Check sheet for the modelled part. Datum: model origin and axes. Units: mm. A direction names the side the tool comes from. Give positions to 0.01 mm unless a question says otherwise; leave off trailing zeros. Order: outer loops, then holes, each group sorted by start corner. A loop starts at its lowest first (then second) coordinate and runs counter-clockwise, first axis right, second up.
from build123d import *

# Parameters (mm, degrees)
SKETCH1_R           = 2
BOSS_EXTRUDE1_DEPTH = 10
CHAMFER2_SIZE       = 10
BOSS_EXTRUDE2_DEPTH = 10
BOSS_EXTRUDE3_DEPTH = 10
SKETCH6_W           = 239.348674296
SKETCH6_H           = 140
BOSS_EXTRUDE4_DEPTH = 10
CUT_EXTRUDE1_DEPTH  = 10
CUT_EXTRUDE2_DEPTH  = 10
CUT_EXTRUDE3_DEPTH  = 10
BOSS_EXTRUDE5_DEPTH = 40
SKETCH13_R          = 10
CUT_EXTRUDE4_DEPTH  = 15
BOSS_EXTRUDE6_DEPTH = 40
SKETCH15_R          = 10
CUT_EXTRUDE5_DEPTH  = 15
BOSS_EXTRUDE7_DEPTH = 40
SKETCH17_R          = 10
CUT_EXTRUDE6_DEPTH  = 15


with BuildPart() as part:
    # Sketch1 → Boss-Extrude1 (new body)
    with BuildSketch(Plane(origin=(0, 0, 0), x_dir=(1, 0, 0), z_dir=(0, 1, 0))):
        Polygon((0, 181.282032303), (-136.994845224, -56), (136.994845224, -56), align=None)
        with Locations(Location((-38.248711306, 59.033320997, 0), (0, 0, 270))):
            Circle(SKETCH1_R, mode=Mode.SUBTRACT)
        with Locations(Location((-50.748711306, 37.382685902, 0), (0, 0, 270))):
            Circle(SKETCH1_R, mode=Mode.SUBTRACT)
        with Locations(Location((37.748711306, 59.899346401, 0), (0, 0, 270))):
            Circle(SKETCH1_R, mode=Mode.SUBTRACT)
        with Locations(Location((50.248711306, 38.248711306, 0), (0, 0, 270))):
            Circle(SKETCH1_R, mode=Mode.SUBTRACT)
        with Locations(Location((-12, -28, 0), (0, 0, 270))):
            Circle(SKETCH1_R, mode=Mode.SUBTRACT)
        with Locations(Location((13, -28, 0), (0, 0, 270))):
            Circle(SKETCH1_R, mode=Mode.SUBTRACT)
    extrude(amount=BOSS_EXTRUDE1_DEPTH)

    # Chamfer2
    chamfer2_edges = [part.edges().sort_by_distance(p)[0] for p in [
        (68.497422612, 0, -62.641016151),
        (-68.497422612, 0, -62.641016151),
        (0, 0, 56),
    ]]
    chamfer(chamfer2_edges, length=CHAMFER2_SIZE - 0.0001)  # a hair under: the kernel refuses the full size

    # Sketch4 → Boss-Extrude2 (add)
    with BuildSketch(Plane(origin=(34.918584287, -40.320508076, -20.160254038), x_dir=(0.7905694150420945, 0.547722557505166, 0.2738612787525844), z_dir=(0.6123724356957949, -0.7071067811865465, -0.3535533905932751))):
        Polygon((107.208489537, 41.143650786), (215.652023231, -47.400123699), (64.274630088, -232.798809596), (-44.168903606, -144.255035111), align=None)
    extrude(amount=BOSS_EXTRUDE2_DEPTH)

    # Sketch5 → Boss-Extrude3 (add)
    with BuildSketch(Plane(origin=(-34.918584287, -40.320508076, -20.160254038), x_dir=(0.7905694150420941, -0.5477225575051675, -0.27386127875258237), z_dir=(-0.6123724356957955, -0.7071067811865476, -0.35355339059327195))):
        Polygon((44.168903606, -144.255035111), (-64.274630088, -232.798809596), (-215.652023231, -47.400123699), (-107.208489537, 41.143650786), align=None)
    extrude(amount=BOSS_EXTRUDE3_DEPTH)

    # Sketch6 → Boss-Extrude4 (add)
    with BuildSketch(Plane(origin=(0, -23, 23), x_dir=(1, 0, 0), z_dir=(0, -0.7071067811865468, 0.7071067811865483))):
        with Locations((0, 102.526911935)):
            Rectangle(SKETCH6_W, SKETCH6_H)
    extrude(amount=BOSS_EXTRUDE4_DEPTH)

    # Sketch8 → Cut-Extrude1 (cut)
    with BuildSketch(Plane(origin=(-34.918584287, -40.320508076, -20.160254038), x_dir=(0.7905694150420941, -0.5477225575051675, -0.2738612787525823), z_dir=(0.6123724356957955, 0.7071067811865477, 0.35355339059327195))):
        Polygon((-33.923185833, 197.463935256), (-49.415119218, 210.113045896), (-115.822950082, 128.780395626), (-84.839083312, 103.482174345), (-18.431252448, 184.814824615), align=None)
    extrude(amount=-CUT_EXTRUDE1_DEPTH, mode=Mode.SUBTRACT)

    # Sketch10 → Cut-Extrude2 (cut)
    with BuildSketch(Plane(origin=(34.918584287, -40.320508076, -20.160254038), x_dir=(0.7905694150420944, 0.5477225575051661, 0.2738612787525847), z_dir=(-0.6123724356957952, 0.7071067811865464, 0.3535533905932753))):
        Polygon((174.960769477, 24.728878015), (190.452702862, 37.377988656), (124.044871998, 118.710638926), (93.061005228, 93.412417645), (159.468836092, 12.079767374), align=None)
    extrude(amount=-CUT_EXTRUDE2_DEPTH, mode=Mode.SUBTRACT)

    # Sketch11 → Cut-Extrude3 (cut)
    with BuildSketch(Plane(origin=(0, -23, 23), x_dir=(1, 0, 0), z_dir=(0, 0.7071067811865468, -0.7071067811865483))):
        Polygon((-111.5, -126.669047558), (-111.5, -146.669047558), (-6.5, -146.669047558), (-6.5, -106.669047558), (-111.5, -106.669047558), align=None)
    extrude(amount=-CUT_EXTRUDE3_DEPTH, mode=Mode.SUBTRACT)

    # Sketch12 → Boss-Extrude5 (add)
    with BuildSketch(Plane(origin=(-34.918584287, -40.320508076, -20.160254038), x_dir=(0.7905694150420941, -0.5477225575051675, -0.2738612787525823), z_dir=(0.6123724356957955, 0.7071067811865477, 0.35355339059327195))):
        Polygon((-18.910434822, 136.793783558), (-24.719909842, 141.537200048), (-43.693575803, 118.299299971), (-32.074625764, 108.81246699), (-13.100959803, 132.050367067), align=None)
    extrude(amount=BOSS_EXTRUDE5_DEPTH)

    # Sketch13 → Cut-Extrude4 (cut)
    with BuildSketch(Plane(origin=(-66.542804663, 76.83701237, -38.418506185), x_dir=(0.7905694150420933, 0.5477225575051691, -0.27386127875258187), z_dir=(-0.6123724356957966, 0.7071067811865475, -0.35355339059327057))):
        with Locations(Location((21.287016809, 84.607785007, 0), (0, 0, 162.976133815))):
            Circle(SKETCH13_R)
    extrude(amount=-CUT_EXTRUDE4_DEPTH, mode=Mode.SUBTRACT)

    # Sketch14 → Boss-Extrude6 (add)
    with BuildSketch(Plane(origin=(34.918584287, -40.320508076, -20.160254038), x_dir=(0.7905694150420944, 0.5477225575051661, 0.2738612787525847), z_dir=(-0.6123724356957952, 0.7071067811865464, 0.3535533905932753))):
        Polygon((112.513853563, 22.15347651), (118.323328583, 26.896893), (99.349662622, 50.134793077), (87.730712583, 40.647960097), (106.704378544, 17.41006002), align=None)
    extrude(amount=BOSS_EXTRUDE6_DEPTH)

    # Sketch15 → Cut-Extrude5 (cut)
    with BuildSketch(Plane(origin=(66.542804663, 76.83701237, -38.418506185), x_dir=(0.7905694150420963, -0.5477225575051645, 0.2738612787525824), z_dir=(0.6123724356957928, 0.7071067811865488, -0.3535533905932746))):
        with Locations(Location((53.342735971, -6.794621963, 0), (0, 0, 197.023866185))):
            Circle(SKETCH15_R)
    extrude(amount=-CUT_EXTRUDE5_DEPTH, mode=Mode.SUBTRACT)

    # Sketch16 → Boss-Extrude7 (add)
    with BuildSketch(Plane(origin=(0, -23, 23), x_dir=(1, 0, 0), z_dir=(0, 0.7071067811865468, -0.7071067811865483))):
        Polygon((-74, -76.669047558), (-74, -84.169047558), (-44, -84.169047558), (-44, -69.169047558), (-74, -69.169047558), align=None)
    extrude(amount=BOSS_EXTRUDE7_DEPTH)

    # Sketch17 → Cut-Extrude6 (cut)
    with BuildSketch(Plane(origin=(0, 59.516504294, 59.516504294), x_dir=(1, 0, 0), z_dir=(0, 0.7071067811865482, 0.7071067811865468))):
        with Locations(Location((-59, -12.526911935, 0), (0, 0, 270))):
            Circle(SKETCH17_R)
    extrude(amount=-CUT_EXTRUDE6_DEPTH, mode=Mode.SUBTRACT)


solid = part.part
1) Material ranges on L1, parallel to X at y = 7, z = 28; L2, parallel to X at y = 43.5, z = -126; L3, parallel to Z at x = -50.5, y = 33, recorded low to high.
Recorded:
L1: x = -133.69 to -14, -10 to 11, 15 to 133.69
L2: x = -86.93 to -70.6, -54.47 to -53.24, -40.48 to -30.24, 70.6 to 86.93
L3: z = -168.1 to -139.81, -137.7 to -111.45, 64.82 to 93.14
2) Section check B-B, the plane z = -72. Record the cut outline in (x, y), then the cut area to 3 significant figures.
Recorded:
outline: (-174.02, 91.92) - (-59.71, -7.07) - (-51.55, 0) - (51.55, 0) - (59.71, -7.07) - (120.25, 45.36) - (112.08, 52.43) - (63.09, 10) - (-63.09, 10) - (-165.86, 98.99) - close; (144.74, 80.71) - (152.91, 73.64) - (174.02, 91.92) - (165.86, 98.99) - close
area: 3,920 mm2
3) Draft check along X on faces 4 (the face through (-2, 0, -36)), 5 (the face through (-44, 45, 63)), 6 (the face through (-128.213, 6.041, 48.708)). Enter one of: +X half, -X half, draft (parallel to the pull), parting line (faces both ways), or undercut.
Recorded:
face 4: undercut
face 5: +X half
face 6: -X half
4) Depth check by flat-ended pin: pin 1 Ø5 at (y, z) = (74, -39) entering from -X; pin 2 Ø2.5 at (x, z) = (-12, 28) entering from -Y; pin 3 Ø3 at (x, z) = (-109.5, -71.5) entering from +Y; pin 4 Ø5 at (y, z) = (68, -73.5) entering from -X. Enter the tip coordinate at first touch or a pass-through.
Recorded:
pin 1: stops at x = -175.6
pin 2: passes through
pin 3: stops at y = 51.44
pin 4: stops at x = -148.76
5) Section check A-A, the plane z = -147.5. Record the cut outline in (x, y), then the cut area to 3 significant figures.
Recorded:
outline: (-130.43, 91.92) - (-109.32, 73.64) - (-101.15, 80.71) - (-122.27, 98.99) - close; (-76.66, 45.36) - (-16.12, -7.07) - (-7.96, 0) - (7.96, 0) - (16.12, -7.07) - (130.43, 91.92) - (122.27, 98.99) - (19.5, 10) - (-19.5, 10) - (-68.49, 52.43) - close
area: 3,050 mm2
6) Set-up check for faces 1 (the face through (62.02, -3.49, -60.84)), 2 (the face through (-44.78, 50.461, -128.865)), 3 (the face through (-74, 45, 63)): record each of +Z, -Z, +X, -X, +Y, -Y from which the full face is reachable in a straight line by a thin tool's end or side.
Recorded:
face 1: -Y
face 2: +Y
face 3: -X, +Y
7) Section check C-C, the plane x = -144.5. Record the cut outline in (y, z).
Recorded:
outline: (14.52, 31.67) - (91.92, -123.13) - (98.99, -108.99) - (28.67, 31.67) - close
